```python
from build123d import *

# Parameters (mm, degrees)
BOSS_EXTRUDE1_DEPTH = 6.35
SKETCH2_R           = 85
CUT_EXTRUDE1_DEPTH  = 6.35
FILLET1_R           = 60
SKETCH3_W           = 6
SKETCH3_H           = 185
CUT_EXTRUDE2_DEPTH  = 6.35
FILLET2_R           = 20


with BuildPart() as part:
    # Sketch1 → Boss-Extrude1 (new body)
    with BuildSketch(Plane(origin=(0, 0, 0), x_dir=(1, 0, 0), z_dir=(0, 1, 0))):
        Polygon((0, 0), (-350, -606.217782649), (350, -606.217782649), align=None)
    extrude(amount=BOSS_EXTRUDE1_DEPTH)

    # Sketch2 → Cut-Extrude1 (cut)
    with BuildSketch(Plane(origin=(0, 6.35, 0), x_dir=(1, 0, 0), z_dir=(0, 1, 0))):
        with Locations((0, -404.145188433)):
            Circle(SKETCH2_R)
    extrude(amount=-CUT_EXTRUDE1_DEPTH, mode=Mode.SUBTRACT)

    # Fillet1
    fillet1_edges = [part.edges().sort_by_distance(p)[0] for p in [
        (350, 3.175, 606.217782649),
        (-350, 3.175, 606.217782649),
        (0, 3.175, 0),
    ]]
    fillet(fillet1_edges, radius=FILLET1_R)

    # Sketch3 → Cut-Extrude2 (cut)
    with BuildSketch(Plane(origin=(0, 6.35, 0), x_dir=(1, 0, 0), z_dir=(0, 1, 0))):
        Polygon((27.480762114, -416.547112221), (24.480762114, -421.743264644), (184.695461814, -514.243264644), (187.695461814, -509.047112221), align=None)
        with Locations((0, -281.645188433)):
            Rectangle(SKETCH3_W, SKETCH3_H)
        Polygon((-24.480762114, -421.743264644), (-27.480762114, -416.547112221), (-187.695461814, -509.047112221), (-184.695461814, -514.243264644), align=None)
    extrude(amount=-CUT_EXTRUDE2_DEPTH, mode=Mode.SUBTRACT)

    # Fillet2
    fillet2_edges = [part.edges().sort_by_distance(p)[0] for p in [
        (3, 3.175, 319.198146106),
        (-3, 3.175, 319.198146106),
        (-75.066296631, 3.175, 444.020633385),
        (-72.066296631, 3.175, 449.216785807),
        (72.066296631, 3.175, 449.216785807),
        (75.066296631, 3.175, 444.020633385),
    ]]
    fillet(fillet2_edges, radius=FILLET2_R)


solid = part.part
```
Geometry: final body of the model. Coordinates: model frame, mm. A direction names the side the tool comes from. Round coordinates to 2 decimals unless told otherwise and drop trailing zeros. Order: outer loops, then holes, each group sorted by start corner. A loop starts at its lowest first (then second) coordinate and runs counter-clockwise, first axis right, second up. Notation, with made-up numbers: (24.5, 78) -> (43.5, 78) arc R31 cw to (43.5, 113) -> close; hole circle Ø8 at (75.5, -4). An arc over 180 degrees is marked (long way). Use CSV: the item, a comma, the result in double quotes. Start each with the question number.
1) Section D-D (z = 145). Return the cut outline in (x, y).
2) Draft query along Z for faces 3 (the face through (-138.278, 3.219, 480.516)), 4 (the face through (-298.473, 3.219, 575.453)), 5 (the face through (-173.28, 3.13, 300.13)). Return one class per face: +Z half, -Z half, draft (parallel to the pull), parting line (faces both ways), or undercut.
3) Set-up query: faces 1 (the face through (-0.88, 3.219, 60.006)), 2 (the face through (-73.12, 3.22, 360.8)). Return all of +Z, -Z, +X, -X, +Y, -Y with unobstructed straight access to the full face (end or side cutting, diameter ignored); none if empty.
4) Section B-B (y = 2.5). Return the cut outline in (x, z), and give its area (3 significant figures).
5) Section C-C (z = 417). Return the cut outline in (x, y).
6) First-contact query: pin 1 Ø3 at (x, y) = (-75, 2) entering from -Z; pin 2 Ø1.9 at (y, z) = (1.5, 244) entering from -X. Flat tips, straight axial feed; report the tip coordinate or a pass-through.
7) Material intervals for line 1 along X through (y, z) = (0.5, 242); line 2 along Z through (x, y) = (45, 2.5); line 3 along X through (y, z) = (0.75, 550.5), sorted ascending. Write a range as from..to.
8) Section A-A (x = 136). Return the cut outline in (y, z), and give its area (3 significant figures).
Returned:
1,outline,"(-83.72, 0) -> (83.72, 0) -> (83.72, 6.35) -> (-83.72, 6.35) -> close"
2,face 3,"undercut"
2,face 4,"parting line"
2,face 5,"-Z half"
3,face 1,"-Z, +Y, -Y"
3,face 2,"+Y, -Y"
4,outline,"(-298.04, 516.22) -> (-51.96, 90) arc R60 ccw to (51.96, 90) -> (298.04, 516.22) arc R60 ccw to (246.08, 606.22) -> (-246.08, 606.22) arc R60 ccw to start; hole (-187.7, 509.05) -> (-90.22, 452.77) arc R20 cw to (-81.13, 429.49) arc R85 ccw to (-18.62, 321.21) arc R20 cw to (-3, 301.7) -> (-3, 189.15) -> (3, 189.15) -> (3, 301.7) arc R20 cw to (18.62, 321.21) arc R85 ccw to (81.13, 429.49) arc R20 cw to (90.22, 452.77) -> (187.7, 509.05) -> (184.7, 514.24) -> (87.22, 457.97) arc R20 cw to (62.51, 461.74) arc R85 ccw to (-62.51, 461.74) arc R20 cw to (-87.22, 457.97) -> (-184.7, 514.24) -> close"
4,area,"179,000 mm²"
5,outline,"(-240.76, 0) -> (-84.02, 0) -> (-84.02, 6.35) -> (-240.76, 6.35) -> close; (84.02, 0) -> (240.76, 0) -> (240.76, 6.35) -> (84.02, 6.35) -> close"
6,pin 1,"stops at z = 127.31"
6,pin 2,"stops at x = -141.42"
7,line 1,"x = -139.72..-3, 3..139.72"
7,line 2,"z = 80.31..332.03, 476.26..606.22"
7,line 3,"x = -305.92..305.92"
8,outline,"(0, 235.56) -> (6.35, 235.56) -> (6.35, 479.2) -> (0, 479.2) -> close; (0, 486.13) -> (6.35, 486.13) -> (6.35, 606.22) -> (0, 606.22) -> close"
8,area,"2,310 mm²"
